Geometry: final body of the model. Coordinates: model frame, mm. A direction names the side the tool comes from. Give positions to 0.01 mm unless a question says otherwise; leave off trailing zeros. Write each loop counter-clockwise with the first axis right and the second up, starting at its lowest first coordinate (ties: lowest second). Pieces come first, ordered by that corner, then holes.
Q1. Mould query, pull axis Y, two halves, no side actions, for faces 3 (the cylindrical face through (-5.199, 21.215, 0.986)), 4 (the flat face through (-2, 19.5, 1)), 5 (the cylindrical face through (-5.215, 14.301, 0.986)). Classes: +Y half, -Y half, draft (parallel to the pull), parting line (faces both ways), or undercut.
Q2. Section B-B (z = 0.9). Return the cut outline in (x, y), plus the area to 3 significant figures.
Q3. Section A-A (x = -3). Return the cut outline in (y, z), plus the area to 3 significant figures.
Q4. Line query: line 1 (X direction, y = 16.5, z = 1.7); line 2 (Y direction, x = 1, z = 1.45); line 3 (X direction, y = 21.25, z = 0.55). Output: solid intervals per line, ascending.
Q5. Reachability of faces 1 (the flat face through (-0.75, 18, 1)), 2 (the flat face through (0, 21.5, 1)) from +Z, -Z, +X, -X, +Y, -Y: full face, straight path, thin tool, end or side. Return the list, or none.
from build123d import *

# Parameters (mm, degrees)
SKETCH1_W           = 2.75
SKETCH1_H           = 3.5
BOSS_EXTRUDE1_DEPTH = 2


with BuildPart() as part:
    # Sketch1 → Boss-Extrude1 (new body)
    with BuildSketch(Plane.XY):
        with BuildLine():
            Line((4.5, 21.5), (-4.5, 21.5))
            ThreePointArc((-4.5, 21.5), (-5.207106781, 21.207106781), (-5.5, 20.5))
            Line((-5.5, 20.5), (-5.5, 15))
            ThreePointArc((-5.5, 15), (-5.207106781, 14.292893219), (-4.5, 14))
            Line((-4.5, 14), (4.5, 14))
            ThreePointArc((4.5, 14), (5.207106781, 14.292893219), (5.5, 15))
            Line((5.5, 15), (5.5, 20.5))
            ThreePointArc((5.5, 20.5), (5.207106781, 21.207106781), (4.5, 21.5))
        make_face()
        with Locations((2.125, 17.75)):
            Rectangle(SKETCH1_W, SKETCH1_H, mode=Mode.SUBTRACT)
        with Locations((-2.125, 17.75)):
            Rectangle(SKETCH1_W, SKETCH1_H, mode=Mode.SUBTRACT)
    extrude(amount=BOSS_EXTRUDE1_DEPTH)


solid = part.part
Computed:
1. face 3: +Y half
1. face 4: undercut
1. face 5: -Y half
2. outline: (-5.5, 15) arc R1 ccw to (-4.5, 14) - (4.5, 14) arc R1 ccw to (5.5, 15) - (5.5, 20.5) arc R1 ccw to (4.5, 21.5) - (-4.5, 21.5) arc R1 ccw to (-5.5, 20.5) - close; hole (-3.5, 16) - (-0.75, 16) - (-0.75, 19.5) - (-3.5, 19.5) - close; hole (0.75, 16) - (3.5, 16) - (3.5, 19.5) - (0.75, 19.5) - close
2. area: 62.4 mm2
3. outline: (14, 0) - (16, 0) - (16, 2) - (14, 2) - close; (19.5, 0) - (21.5, 0) - (21.5, 2) - (19.5, 2) - close
3. area: 8.00 mm2
4. line 1: x = -5.5 to -3.5, -0.75 to 0.75, 3.5 to 5.5
4. line 2: y = 14 to 16, 19.5 to 21.5
4. line 3: x = -5.16 to 5.16
5. face 1: +Z, -Z
5. face 2: +Z, -Z, +X, -X, +Y
